Source: CAD feature listing. Evaluate the final solid. Frame: model axes, mm. Give positions to 0.01 mm unless a question says otherwise; leave off trailing zeros. Order: outer loops, then holes, each group sorted by start corner. A loop starts at its lowest first (then second) coordinate and runs counter-clockwise, first axis right, second up. Notation, with made-up numbers: M 18,62.25 L 51,62.25 A24 cw 51,72.25 Z; hole C 24,-20 d2. An arc over 180 degrees is marked long. Answer as a JSON object with one key per item and string values. Group by question number.
1. Section query B-B (z = -1.8). Output: boundary loops of the cut face in (x, y) (3 decimals).
2. Section query A-A (y = 0). Output: boundary loops of the cut face in (x, z) (3 decimals).
3. Section query C-C (x = -43.18). Output: boundary loops of the cut face in (y, z) (3 decimals), plus the area to 3 significant figures.
4. Material intervals for L1, parallel to Y at x = -12.7, z = -1.25 (3 decimals); L2, parallel to Y at x = 43.18, z = -1.65; L3, parallel to X at y = 0, z = -1, sorted ascending. Write a range as [from, to].
5. Pull-direction query (Y, two-part tool) for faces 1 (the flat face through (1, 38.1, -2)), 2 (the flat face through (-50.8, 1, -2)), 3 (the cylindrical face through (-12.812, -19.687, -1.61)); classes: +Y half, -Y half, draft (parallel to the pull), parting line (faces both ways), or undercut.
6. Section query D-D (x = -12.7). Output: boundary loops of the cut face in (y, z) (3 decimals), plus the area to 3 significant figures.
Autodesk Inventor part; units mm, degrees
ref_plane "YZ Plane" through (0, 0, 0) normal (1, 0, 0) x (0, 1, 0)
ref_plane "XZ Plane" through (0, 0, 0) normal (0, 1, 0) x (-1, 0, 0)
ref_plane "XY Plane" through (0, 0, 0) normal (0, 0, 1) x (1, 0, 0)
sketch "Sketch1" plane through (0, 0, 0) normal (0, 0, 1) x (1, 0, 0)
  line L0 (-50.8, -38.1) -> (50.8, -38.1)
  line L1 (50.8, -38.1) -> (50.8, 38.1)
  line L2 (50.8, 38.1) -> (-50.8, 38.1)
  line L3 (-50.8, 38.1) -> (-50.8, -38.1)
  line L4 (-50.8, -38.1) -> (50.8, 38.1) construction
  line L5 (50.8, -38.1) -> (-50.8, 38.1) construction
  point P0 (0, 0)
  dimension "d0" = 101.6
  dimension "d1" = 76.2
extrude "Extrusion1" add sketch "Sketch1" against normal blind 3.175
sketch "Sketch2" plane through (0, 0, 0) normal (0, 0, 1) x (1, 0, 0)
  circle A0 centre (43.18, 0) radius 2.54
  line L0 (50.8, -38.1) -> (50.8, 38.1)
  line L1 (0, 38.1) -> (0, -38.1) construction
  circle A1 centre (-43.18, 0) radius 2.54
  point P0 (0, 0)
  dimension "d4" = 5.08
  dimension "d5" = 7.62
hole "Hole1" at (-43.18, 0, 0) at (43.18, 0, 0) direction (0, 0, -1) diameter 5.08 end through all
sketch "Sketch3" plane through (0, 0, 0) normal (0, 0, 1) x (1, 0, 0)
  line L0 (0, 29.2764) -> (0, -24.7835) construction
  line L1 (50.8, 38.1) -> (-50.8, 38.1) construction
  line L2 (-18.9862, 0) -> (21.3051, 0) construction
  point P0 (0, 0)
  point P1 (-12.7, 22.225)
  point P2 (0, 38.1)
  point P3 (12.7, 22.225)
  point P4 (-12.7, -22.225)
  point P5 (12.7, -22.225)
  dimension "d13" = 22.225
  dimension "d14" = 12.7
hole "Hole2" at (-12.7, 22.225, 0) at (12.7, 22.225, 0) at (-12.7, -22.225, 0) at (12.7, -22.225, 0) direction (0, 0, -1) diameter 5.08 end through all
properties part number "VEX Motor Mount" material "Aluminum 6061"
Answer sheet:
{
 "1": {"outline": "M -50.8,-38.1 L 50.8,-38.1 L 50.8,38.1 L -50.8,38.1 Z; hole C -43.18,0 d5.08; hole C -12.7,-22.225 d5.08; hole C -12.7,22.225 d5.08; hole C 12.7,-22.225 d5.08; hole C 12.7,22.225 d5.08; hole C 43.18,0 d5.08"},
 "2": {"outline": "M -50.8,-3.175 L -45.72,-3.175 L -45.72,0 L -50.8,0 Z; M -40.64,-3.175 L 40.64,-3.175 L 40.64,0 L -40.64,0 Z; M 45.72,-3.175 L 50.8,-3.175 L 50.8,0 L 45.72,0 Z"},
 "3": {"outline": "M -38.1,-3.175 L -2.54,-3.175 L -2.54,0 L -38.1,0 Z; M 2.54,-3.175 L 38.1,-3.175 L 38.1,0 L 2.54,0 Z", "area": "226 mm^2"},
 "4": {"L1": "[-38.1, -24.765], [-19.685, 19.685], [24.765, 38.1]", "L2": "[-38.1, -2.54], [2.54, 38.1]", "L3": "[-50.8, -45.72], [-40.64, 40.64], [45.72, 50.8]"},
 "5": {"face 1": "+Y half", "face 2": "draft", "face 3": "undercut"},
 "6": {"outline": "M -38.1,-3.175 L -24.765,-3.175 L -24.765,0 L -38.1,0 Z; M -19.685,-3.175 L 19.685,-3.175 L 19.685,0 L -19.685,0 Z; M 24.765,-3.175 L 38.1,-3.175 L 38.1,0 L 24.765,0 Z", "area": "210 mm^2"}
}
